Read the model definition and answer for the solid it produces. Units are mm, in the model's axes. A direction names the side the tool comes from. Coordinates: 2 decimals unless noted, no trailing zeros. Order: outer loops, then holes, each group sorted by start corner. A loop starts at its lowest first (then second) coordinate and runs counter-clockwise, first axis right, second up. Notation, with made-up numbers: M 54,73 L 94,73 A14 ccw 94,80 Z; hole C 26.5,-36 d2. An arc over 180 degrees is marked long. Put each result on its own line as item: value.
from build123d import *

# Parameters (mm, degrees)
F0_W     = 206
F0_H     = 81
F1_DEPTH = 41.68
F2_R     = 2.65
F3_DEPTH = 10
F4_W     = 50
F4_H     = 20
F5_DEPTH = 25


with BuildPart() as f1:
    # F0 (on Front) → F1 (new body)
    with BuildSketch(Plane.XZ):
        Rectangle(F0_W, F0_H)
    extrude(amount=F1_DEPTH)

    # F2 (on face) → F3 (cut)
    with BuildSketch(Plane(origin=(0, 0, 0), x_dir=(-1, 0, 0), z_dir=(0, 1, 0))):
        with Locations((-81, 36.75)):
            Circle(F2_R)
        with Locations((-81, -36.75)):
            Circle(F2_R)
        with Locations((81, -36.75)):
            Circle(F2_R)
        with Locations((81, 36.75)):
            Circle(F2_R)
    extrude(amount=-F3_DEPTH, mode=Mode.SUBTRACT)

    # F4 (on face) → F5 (join)
    with BuildSketch(Plane(origin=(0, 0, 0), x_dir=(-1, 0, 0), z_dir=(0, 1, 0))):
        with Locations((0, -20.5)):
            Rectangle(F4_W, F4_H)
    extrude(amount=F5_DEPTH)


solid = f1.part
Q1. Find section D-D on z = -18. Write down the section's boundary in (x, y), plus the area to 3 significant figures.
Answers below:
outline: M -103,-41.68 L 103,-41.68 L 103,0 L 25,0 L 25,25 L -25,25 L -25,0 L -103,0 Z
area: 9,840 mm^2
Q2. Find section C-C on y = 8. Write down the section's boundary in (x, z), plus the area to 3 significant figures.
Answers below:
outline: M -25,-30.5 L 25,-30.5 L 25,-10.5 L -25,-10.5 Z
area: 1,000 mm^2
Q3. Consider line 1 along Z through (x, y) = (81, -6.75); line 2 along X through (y, z) = (-4, -36); line 3 along X through (y, z) = (14, -26). Determine where each line is inside the solid, lowest interval first.
Answers below:
line 1: z = -40.5 to -39.4, -34.1 to 34.1, 39.4 to 40.5
line 2: x = -103 to -83.54, -78.46 to 78.46, 83.54 to 103
line 3: x = -25 to 25
Q4. Find section A-A on x = 81. Write down the section's boundary in (y, z).
Answers below:
outline: M -41.68,-40.5 L 0,-40.5 L 0,-39.4 L -10,-39.4 L -10,-34.1 L 0,-34.1 L 0,34.1 L -10,34.1 L -10,39.4 L 0,39.4 L 0,40.5 L -41.68,40.5 Z
Q5. A tool of negligible diameter and unlimited length cuts with its end or side. For faces 1 (the face through (81, -10, 37)), 2 (the face through (0, 12, -10.5)), 3 (the face through (-25, 12, -21)), 4 (the face through (0, 12, -30.5)), from which of +Z, -Z, +X, -X, +Y, -Y can it reach the whole face along a straight path? Write none if from no direction.
Answers below:
face 1: +Y
face 2: +Z, +X, -X, +Y
face 3: +Z, -Z, -X, +Y
face 4: -Z, +X, -X, +Y
Q6. Given pin 1 (6 mm diameter, centred on y = 18.5, z = -16.5, fed in from +X); pin 2 (1 mm diameter, centred on x = 52.5, z = -10.5, fed in from +Y); pin 3 (6 mm diameter, centred on y = 16, z = -18, fed in from -X), each flat-ended and moving along its own axis, determine where each tip first touches the part or whether it passes through.
Answers below:
pin 1: stops at x = 25
pin 2: stops at y = 0
pin 3: stops at x = -25
Q7. Find section B-B on z = -36.75. Write down the section's boundary in (x, y).
Answers below:
outline: M -103,-41.68 L 103,-41.68 L 103,0 L 83.65,0 L 83.65,-10 L 78.35,-10 L 78.35,0 L -78.35,0 L -78.35,-10 L -83.65,-10 L -83.65,0 L -103,0 Z
Q8. For a pull along Z with two mould halves and no side action, classify faces 5 (the face through (-1, -21, -40.5)), 6 (the face through (25, 12, -21)), 7 (the face through (-80.66, -4.93, -34.12)) as +Z half, -Z half, draft (parallel to the pull), parting line (faces both ways), or undercut.
Answers below:
face 5: -Z half
face 6: draft
face 7: undercut
